Source: CAD feature listing. Evaluate the final solid. Frame: model axes, mm. A direction names the side the tool comes from. Round coordinates to 2 decimals unless told otherwise and drop trailing zeros. Write each loop counter-clockwise with the first axis right and the second up, starting at its lowest first coordinate (ties: lowest second). Pieces come first, ordered by that corner, then holes. Notation, with made-up numbers: (29, 72) -> (72, 72) arc R22 ccw to (72, 103) -> close; hole circle Ø3 at (20.5, -28.5). An arc over 180 degrees is marked (long way). Put each result on its own line as item: value.
```python
from build123d import *

# Parameters (mm, degrees)
F0_R     = 14
F0_R_2   = 1.6
F0_R_3   = 4
F0_R_4   = 2.5
F1_DEPTH = 20
F2_DEPTH = 32
F3_DEPTH = 2
F4_START = 5
F4_DEPTH = 15
F5_SIZE2 = 3
F5_SIZE  = 6
F6_R     = 2.5


with BuildPart() as f1:
    # F0 (on Top) → F1 (new body)
    with BuildSketch(Plane.XY):
        Circle(F0_R)
        with Locations((0, -8)):
            Circle(F0_R_2, mode=Mode.SUBTRACT)
        with Locations((-9.5, 0)):
            Circle(F0_R_2, mode=Mode.SUBTRACT)
        Circle(F0_R_3, mode=Mode.SUBTRACT)
        with Locations((9.5, 0)):
            Circle(F0_R_2, mode=Mode.SUBTRACT)
        with Locations((0, 8)):
            Circle(F0_R_2, mode=Mode.SUBTRACT)
        Circle(F0_R_3)
        Circle(F0_R_4, mode=Mode.SUBTRACT)
        Circle(F0_R_4)
    extrude(amount=F1_DEPTH)

    # F0 (on Top) → F2 (join)
    with BuildSketch(Plane.XY):
        Circle(F0_R_4)
    extrude(amount=F2_DEPTH)

    # F0 (on Top) → F3 (join)
    with BuildSketch(Plane.XY):
        Circle(F0_R_3)
        Circle(F0_R_4, mode=Mode.SUBTRACT)
        Circle(F0_R_4)
    extrude(amount=-F3_DEPTH)

    # F0 (on Top) → F4 (join)
    with BuildSketch(Plane.XY.offset(F4_START)):
        with Locations((0, 8)):
            Circle(F0_R_2)
        with Locations((9.5, 0)):
            Circle(F0_R_2)
        with Locations((0, -8)):
            Circle(F0_R_2)
        with Locations((-9.5, 0)):
            Circle(F0_R_2)
    extrude(amount=F4_DEPTH)

    # F5
    f5_edges = [f1.edges().sort_by_distance(p)[0] for p in [
        (-14, 0, 20),
    ]]
    f5_side = f1.faces().sort_by_distance((-13.60402, 0, 20))[0]
    chamfer(f5_edges, length=F5_SIZE, length2=F5_SIZE2, reference=f5_side)

    # F6
    f6_edges = [f1.edges().sort_by_distance(p)[0] for p in [
        (11, 0, 18.5),
        (-8, 0, 20),
        (-14, 0, 17),
        (14, 0, 8.5),
        (-14, 0, 0),
    ]]
    fillet(f6_edges, radius=F6_R)


solid = f1.part
```
Q1. Material intervals for line 1 (Y direction, x = 0, z = 3.9); line 2 (Z direction, x = -6.5, y = -1.25); line 3 (Y direction, x = -1, z = 3.5), sorted ascending. Write a range as [from, to].
Ans:
line 1: y = [-14, -9.6], [-6.4, 6.4], [9.6, 14]
line 2: z = [0, 20]
line 3: y = [-13.96, -9.25], [-6.75, 6.75], [9.25, 13.96]
Q2. Cut plane A-A on z = 22.5. Output: boundary loops of the cut face in (x, y).
Ans:
outline: circle Ø5 at (0, 0)
Q3. Pin query (flat end, axial travel): pin 1 (1 mm diameter, centred on x = 10, y = 0.5, fed in from -Z); pin 2 (2 mm diameter, centred on y = -5.5, z = 13.5, fed in from +X); pin 3 (6 mm diameter, centred on x = -2.5, y = 7.5, fed in from +Z). Return the tip coordinate at first contact, or that it passes through.
Ans:
pin 1: stops at z = 5
pin 2: stops at x = 13.26
pin 3: stops at z = 20
Q4. Reachability of faces 1 (the flat face through (0, 0, 32)), 2 (the flat face through (3, 0, 20)), 3 (the cylindrical face through (-0.35, 6.44, 2.46)) from +Z, -Z, +X, -X, +Y, -Y: full face, straight path, thin tool, end or side. Return the list, or none.
Ans:
face 1: +Z, +X, -X, +Y, -Y
face 2: +Z
face 3: -Z
Q5. Draft query along X for faces 4 (the flat face through (5, 0, 0)), 5 (the flat face through (9, 0, 5)), 6 (the cylindrical face through (-0.54, -2.44, 25.92)). Return one class per face: +X half, -X half, draft (parallel to the pull), parting line (faces both ways), or undercut.
Ans:
face 4: draft
face 5: undercut
face 6: parting line
